from build123d import *

# Parameters (mm, degrees)
SKETCH1_R           = 75.946
BOSS_EXTRUDE1_DEPTH = 12.7
SKETCH2_R           = 69.85
CUT_EXTRUDE1_DEPTH  = 6.35
SKETCH3_R           = 5.35813
SKETCH3_R_2         = 8.2499962
SKETCH3_R_3         = 2.5527
SKETCH3_R_4         = 1.7272
CUT_EXTRUDE2_DEPTH  = 108.59141384
CIRPATTERN1_COUNT   = 4


with BuildPart() as part:
    # Sketch1 → Boss-Extrude1 (new body)
    with BuildSketch(Plane.XY):
        Circle(SKETCH1_R)
    extrude(amount=BOSS_EXTRUDE1_DEPTH)

    # Sketch2 → Cut-Extrude1 (cut)
    with BuildSketch(Plane.XY.offset(12.7)):
        Circle(SKETCH2_R)
    extrude(amount=-CUT_EXTRUDE1_DEPTH, mode=Mode.SUBTRACT)

    # Sketch3 → Cut-Extrude2 (cut, through all)
    with BuildSketch(Plane.XY.offset(6.35)):
        Circle(SKETCH3_R)
        with Locations((-19.05, -32.995567884)):
            Circle(SKETCH3_R_2)
        with Locations((-61.336289969, 16.435009364)):
            Circle(SKETCH3_R_3)
        with Locations((61.336289969, -16.435009364)):
            Circle(SKETCH3_R_3)
        with Locations((44.901280605, 44.901280605)):
            Circle(SKETCH3_R_4)
        with Locations((-44.901280605, 44.901280605)):
            Circle(SKETCH3_R_4)
        with Locations((-44.901280605, -44.901280605)):
            Circle(SKETCH3_R_4)
        with Locations((44.901280605, -44.901280605)):
            Circle(SKETCH3_R_4)
    extrude(amount=-CUT_EXTRUDE2_DEPTH, mode=Mode.SUBTRACT)

    # Sketch5 → CSK for #10 Flat Head Machine Screw (100)1 (revolve, cut)
    with BuildSketch(Plane(origin=(0, 75.946, 6.35), x_dir=(0, 0, 1), z_dir=(1, 0, 0))):
        Polygon((0, 0), (0, 19.05), (2.5527, 17.516183098), (2.5527, 1.960808018), (4.8895, 0), align=None)
    csk_for_10_flat_head_machine_screw_100 = revolve(axis=Axis((0, 82.296, 6.35), (0, -1, 0)), mode=Mode.SUBTRACT)

    # CirPattern1: CSK for #10 Flat Head Machine Screw (100)1 ×4 about axis
    cirpattern1_axis = Axis((0, 0, 12.7), (0, 0, 1))
    for i in range(1, CIRPATTERN1_COUNT):
        add(csk_for_10_flat_head_machine_screw_100.rotate(cirpattern1_axis, i * 360 / CIRPATTERN1_COUNT), mode=Mode.SUBTRACT)


solid = part.part
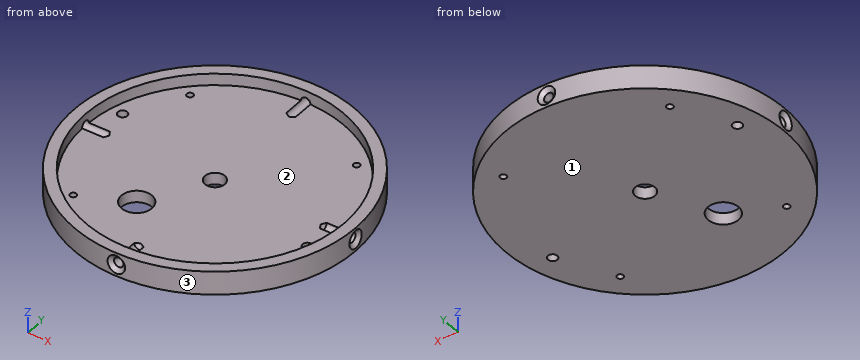
Input: part model. Units: mm. Frame: model coordinates. Face numbers are marked on the shaded views. Coordinates: 2 decimals unless noted, no trailing zeros. Loops run counter-clockwise (first coordinate to the right, second up) from the corner with the lowest first, then second, coordinate; pieces in that order, holes last.
(1) Material intervals for probe 1 along Y at (x, z) = (-45.5, 5.75); probe 2 along Z at (x, y) = (14, -26); probe 3 along Y at (x, z) = (29, 10), sorted ascending.
(2) Section A-A on y = 0. Return the cut outline in (x, z).
(3) Pull-direction query (X, two-part tool) for the marked faces 1, 2 and 3; classes: released by +X, released by -X, zero draft, split by the parting line, or undercut.
(4) First-contact query: pin 1 Ø3 at (x, y) = (49, 15.5) entering from +Z; pin 2 Ø4.5 at (y, z) = (0, 6.35) entering from -X; pin 3 Ø3 at (x, y) = (-44.9, -44.9) entering from +Z; pin 4 Ø5 at (x, z) = (-35.5, 2.5) entering from +Y. Flat tips, straight axial feed; report the tip coordinate or a pass-through.
(5) Section C-C on x = -19.05. Return the cut outline in (y, z), then the cut area to 3 significant figures.
(6) Section D-D on y = 62.5. Return the cut outline in (x, z), then the cut area to 3 significant figures.
Data:
1. probe 1: y = -60.81 to -46.52, -43.28 to 43.28, 46.52 to 60.81
1. probe 2: z = 0 to 6.35
1. probe 3: y = -70.19 to -63.55, 63.55 to 70.19
2. outline: (-75.95, 0) - (-5.36, 0) - (-5.36, 6.35) - (-56.9, 6.35) - (-58.43, 3.8) - (-73.99, 3.8) - (-75.95, 1.46) - close; (-75.95, 11.24) - (-73.99, 8.9) - (-69.85, 8.9) - (-69.85, 12.7) - (-75.95, 12.7) - close; (5.36, 0) - (75.95, 0) - (75.95, 1.46) - (73.99, 3.8) - (58.43, 3.8) - (56.9, 6.35) - (5.36, 6.35) - close; (69.85, 8.9) - (73.99, 8.9) - (75.95, 11.24) - (75.95, 12.7) - (69.85, 12.7) - close
3. face 1: zero draft
3. face 2: undercut
3. face 3: split by the parting line
4. pin 1: stops at z = 6.35
4. pin 2: stops at x = -58.25
4. pin 3: passes through
4. pin 4: stops at y = 68.4
5. outline: (-73.52, 0) - (-41.25, 0) - (-41.25, 6.35) - (-67.2, 6.35) - (-67.2, 12.7) - (-73.52, 12.7) - close; (-24.75, 0) - (73.52, 0) - (73.52, 12.7) - (67.2, 12.7) - (67.2, 6.35) - (-24.75, 6.35) - close
5. area: 909 mm2
6. outline: (-43.15, 0) - (43.15, 0) - (43.15, 12.7) - (31.19, 12.7) - (31.19, 6.35) - (2.55, 6.35) arc R2.55 cw to (-2.55, 6.35) - (-31.19, 6.35) - (-31.19, 12.7) - (-43.15, 12.7) - close
6. area: 690 mm2
